Could you check a few things on this model? Use its own coordinates, in mm. Coordinates: 2 decimals unless noted, no trailing zeros. Loops run counter-clockwise (first coordinate to the right, second up) from the corner with the lowest first, then second, coordinate; pieces in that order, holes last. Notation, with made-up numbers: (33.5, 86.5) - (54.5, 86.5) arc R17 cw to (54.5, 91.5) - close; hole circle Ø8 at (65.25, 69). An arc over 180 degrees is marked (long way). Put each result on its own line as item: value. Start each with the question number.
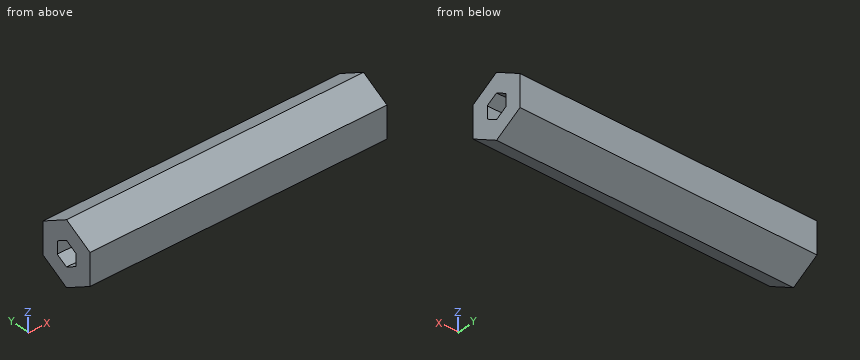
Autodesk Inventor part; units mm, degrees
ref_plane "YZ Plane" through (0, 0, 0) normal (1, 0, 0) x (0, 1, 0)
ref_plane "XZ Plane" through (0, 0, 0) normal (0, 1, 0) x (-1, 0, 0)
ref_plane "XY Plane" through (0, 0, 0) normal (0, 0, 1) x (1, 0, 0)
sketch "Sketch1" plane through (0, 0, 0) normal (1, 0, 0) x (0, 1, 0)
  line L0 (-6.35, -3.6662) -> (0, -7.3323)
  line L1 (-6.35, 3.6662) -> (-6.35, -3.6662)
  line L2 (0, 7.3323) -> (-6.35, 3.6662)
  line L3 (6.35, 3.6662) -> (0, 7.3323)
  line L4 (6.35, -3.6662) -> (6.35, 3.6662)
  line L5 (0, -7.3323) -> (6.35, -3.6662)
  line L6 (2.5, -1.4434) -> (0, -2.8868)
  line L7 (0, -2.8868) -> (-2.5, -1.4434)
  line L8 (-2.5, -1.4434) -> (-2.5, 1.4434)
  line L9 (-2.5, 1.4434) -> (0, 2.8868)
  line L10 (0, 2.8868) -> (2.5, 1.4434)
  line L11 (2.5, 1.4434) -> (2.5, -1.4434)
  point P0 (0, 0)
  point P1 (0, 0)
  dimension "d0" = 5
extrude "Extrusion1" add sketch "Sketch1" along normal blind 69.0855
properties part number "500H x 50mm"
(1) I want a section at A-A on x = 26. List the corners of the cut face in (y, z) for me.
(2) For pin 1 Ø2 at (x, y) = (61.5, -2) entering from +Z; pin 2 Ø3 at (x, y) = (54, -2) entering from +Z, each with a flat end and sliding along its axis, tell me the tip position at first contact or that it passes through.
(3) I want a section at B-B on y = -1. List the corners of the cut face in (x, z) for me.
(4) I want a section at D-D on z = 6. List the corners of the cut face in (x, y) for me.
(5) I need wall thicknesses on L1, parallel to Y at x = 63, z = 1; L2, parallel to Z at x = 57.5, y = 0; L3, parallel to Z at x = 60.5, y = -1.5. Which ranges of each line are inside material? Lowest first, please. Write a range as [from, to].
(6) I want a section at C-C on z = -2.25. List the corners of the cut face in (x, y) for me, and give its area (3 significant figures).
Answer sheet:
1. outline: (-6.35, -3.67) - (0, -7.33) - (6.35, -3.67) - (6.35, 3.67) - (0, 7.33) - (-6.35, 3.67) - close; hole (-2.5, -1.44) - (0, -2.89) - (2.5, -1.44) - (2.5, 1.44) - (0, 2.89) - (-2.5, 1.44) - close
2. pin 1: stops at z = 6.75
2. pin 2: stops at z = 7.04
3. outline: (0, -6.75) - (69.09, -6.75) - (69.09, -2.31) - (0, -2.31) - close; (0, 2.31) - (69.09, 2.31) - (69.09, 6.75) - (0, 6.75) - close
4. outline: (0, -2.31) - (69.09, -2.31) - (69.09, 2.31) - (0, 2.31) - close
5. L1: y = [-6.35, -2.5], [2.5, 6.35]
5. L2: z = [-7.33, -2.89], [2.89, 7.33]
5. L3: z = [-6.47, -2.02], [2.02, 6.47]
6. outline: (0, -6.35) - (69.09, -6.35) - (69.09, -1.1) - (0, -1.1) - close; (0, 1.1) - (69.09, 1.1) - (69.09, 6.35) - (0, 6.35) - close
6. area: 725 mm^2
